Geometry: final body of the model. Coordinates: model frame, mm. Face numbers are marked on the shaded views. Coordinates: 2 decimals unless noted, no trailing zeros. Order: outer loops, then holes, each group sorted by start corner. A loop starts at its lowest first (then second) coordinate and runs counter-clockwise, first axis right, second up. Notation, with made-up numbers: (-4, 23.25) - (27, 23.25) arc R33 cw to (27, 52.25) - close; hole circle Ø1 at (-35, -1). An arc over 180 degrees is marked (long way). Use one line per item in the form item = value. Start each with the question number.
```python
from build123d import *

# Parameters (mm, degrees)
SKETCH1_W           = 50.8
SKETCH1_H           = 31.75
SKETCH1_R           = 4.5593
BOSS_EXTRUDE1_DEPTH = 6.35
SKETCH1_3_R         = 4.5593
SKETCH1_3_R_2       = 2.2479
BOSS_EXTRUDE2_DEPTH = 2.3368


with BuildPart() as part:
    # Sketch1 → Boss-Extrude1 (new body)
    with BuildSketch(Plane(origin=(0, 0, 0), x_dir=(1, 0, 0), z_dir=(0, 1, 0))):
        Rectangle(SKETCH1_W, SKETCH1_H)
        with Locations(Location((0, 0, 0), (0, 0, 270))):
            Circle(SKETCH1_R, mode=Mode.SUBTRACT)
    extrude(amount=BOSS_EXTRUDE1_DEPTH)

    # Sketch1_3 → Boss-Extrude2 (add)
    with BuildSketch(Plane(origin=(0, 0, 0), x_dir=(1, 0, 0), z_dir=(0, 1, 0))):
        with Locations(Location((0, 0, 0), (0, 0, 270))):
            Circle(SKETCH1_3_R)
        with Locations(Location((0, 0, 0), (0, 0, 270))):
            Circle(SKETCH1_3_R_2, mode=Mode.SUBTRACT)
    extrude(amount=BOSS_EXTRUDE2_DEPTH)


solid = part.part
```
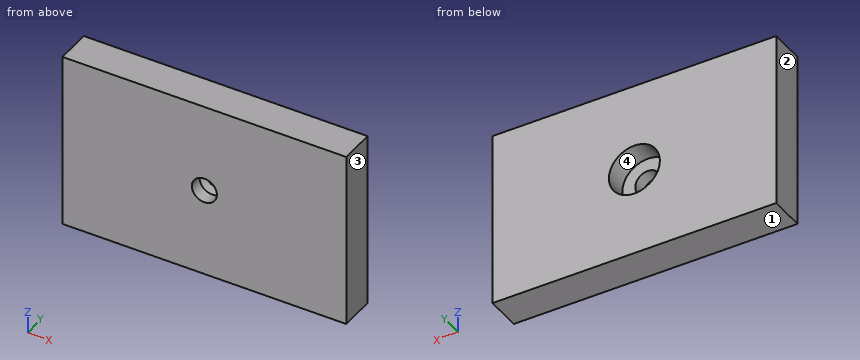
(1) Contact query for flat-ended pins moving along their axis: pin 1 Ø6 at (x, z) = (15.5, 6.5) entering from -Y; pin 2 Ø7.5 at (x, z) = (0, 0) entering from +Y. Output: stop coordinate, or through.
(2) Draft query along X for the marked faces 1, 2, 3 and 4. Return one class per face: released by +X, released by -X, zero draft, split by the parting line, or undercut.
(3) Cut plane A-A on z = 0. Return the cut outline in (x, y).
(4) Cut plane D-D on z = -3.5. Return the cut outline in (x, y).
(5) Material intervals for L1, parallel to X at y = 0.7, z = 0; L2, parallel to X at y = 4.25, z = 0; L3, parallel to Y at x = -1, z = -3.5, sorted ascending. Write a range as from..to.
(6) Cut plane B-B on x = 0. Return the cut outline in (y, z) (3 decimals).
(7) Cut plane C-C on y = 3. Return the cut outline in (x, z) (3 decimals).
Check sheet entries:
q1.pin_1 = 0
q1.pin_2 = 2.34
q2.face_1 = zero draft
q2.face_2 = released by -X
q2.face_3 = released by +X
q2.face_4 = undercut
q3.outline = (-25.4, 0) - (-2.25, 0) - (-2.25, 2.34) - (-4.56, 2.34) - (-4.56, 6.35) - (-25.4, 6.35) - close; (2.25, 0) - (25.4, 0) - (25.4, 6.35) - (4.56, 6.35) - (4.56, 2.34) - (2.25, 2.34) - close
q4.outline = (-25.4, 0) - (25.4, 0) - (25.4, 6.35) - (2.92, 6.35) - (2.92, 2.34) - (-2.92, 2.34) - (-2.92, 6.35) - (-25.4, 6.35) - close
q5.L1 = -25.4..-2.25, 2.25..25.4
q5.L2 = -25.4..-4.56, 4.56..25.4
q5.L3 = 0..2.34
q6.outline = (0, -15.875) - (6.35, -15.875) - (6.35, -4.559) - (2.337, -4.559) - (2.337, -2.248) - (0, -2.248) - close; (0, 2.248) - (2.337, 2.248) - (2.337, 4.559) - (6.35, 4.559) - (6.35, 15.875) - (0, 15.875) - close
q7.outline = (-25.4, -15.875) - (25.4, -15.875) - (25.4, 15.875) - (-25.4, 15.875) - close; hole circle Ø9.119 at (0, 0)
